```python
from build123d import *

# Parameters (mm, degrees)
SKETCH3_R           = 24
BOSS_EXTRUDE1_DEPTH = 19
BOSS_EXTRUDE2_DEPTH = 19
SKETCH7_R           = 8
BOSS_EXTRUDE3_DEPTH = 22.5
BOSS_EXTRUDE4_DEPTH = 26
SKETCH9_W           = 3
SKETCH9_H           = 19.17
BOSS_EXTRUDE5_DEPTH = 3.1
SKETCH10_R          = 1.68
CUT_EXTRUDE1_DEPTH  = 15
SKETCH11_R          = 21.7
CUT_EXTRUDE2_DEPTH  = 2
SKETCH12_R          = 12.95
SKETCH12_R_2        = 10.35
BOSS_EXTRUDE6_DEPTH = 2.06
SKETCH13_R          = 3.35
BOSS_EXTRUDE7_DEPTH = 10
BOSS_EXTRUDE8_DEPTH = 6.5


with BuildPart() as part:
    # Sketch3 → Boss-Extrude1 (new body)
    with BuildSketch(Plane.XY):
        with Locations((225, 142.5)):
            Circle(SKETCH3_R)
    extrude(amount=BOSS_EXTRUDE1_DEPTH)

    # Sketch5 → Boss-Extrude2 (add)
    with BuildSketch(Plane.XY):
        with BuildLine():
            Line((201, 142.5), (200.127626755, 106.785172639))
            Line((200.127626755, 106.785172639), (203.414220338, 106.785172639))
            Line((203.414220338, 106.785172639), (215.733540757, 120.361058447))
            ThreePointArc((215.733540757, 120.361058447), (205.020072299, 129.203290291), (201, 142.5))
        make_face()
    extrude(amount=BOSS_EXTRUDE2_DEPTH)

    # Sketch7 → Boss-Extrude3 (add)
    with BuildSketch(Plane(origin=(0, 128.5, 0), x_dir=(-1, 0, 0), z_dir=(0, -1, 0))):
        with Locations(Location((-233.969805688, -10, 0), (0, 0, 270))):
            Circle(SKETCH7_R)
    extrude(amount=BOSS_EXTRUDE3_DEPTH)

    # Sketch8 → Boss-Extrude4 (add)
    with BuildSketch(Plane(origin=(0, 158.5, 0), x_dir=(-1, 0, 0), z_dir=(0, -1, 0))):
        Polygon((-241.33102162, -5.75), (-241.33102162, -14.25), (-233.969805688, -18.5), (-226.608589756, -14.25), (-226.608589756, -5.75), (-233.969805688, -1.5), align=None)
    extrude(amount=-BOSS_EXTRUDE4_DEPTH)

    # Sketch9 → Boss-Extrude5 (add)
    with BuildSketch(Plane(origin=(197.401507206, -4.821745091, 0), x_dir=(0, 0, 1), z_dir=(-0.999701816720525, 0.024418796974499463, 0))):
        with Locations((20.5, 121.225206973)):
            Rectangle(SKETCH9_W, SKETCH9_H)
    extrude(amount=-BOSS_EXTRUDE5_DEPTH)

    # Sketch10 → Cut-Extrude1 (cut)
    with BuildSketch(Plane(origin=(197.401507206, -4.821745091, 0), x_dir=(0, 0, 1), z_dir=(-0.9997018167205249, 0.02441879697449946, 0))):
        with Locations(Location((3.14, 143.570206973, 0), (0, 0, 270))):
            Circle(SKETCH10_R)
        with BuildLine():
            Line((0, 119.880206973), (0, 115.990206973))
            Line((0, 115.990206973), (3.205, 115.990206973))
            ThreePointArc((3.205, 115.990206973), (5.15, 117.935206973), (3.205, 119.880206973))
            Line((3.205, 119.880206973), (0, 119.880206973))
        make_face()
        with BuildLine():
            Line((22, 115.990206973), (22, 119.880206973))
            Line((22, 119.880206973), (18.795, 119.880206973))
            ThreePointArc((18.795, 119.880206973), (16.85, 117.935206973), (18.795, 115.990206973))
            Line((18.795, 115.990206973), (22, 115.990206973))
        make_face()
    extrude(amount=-CUT_EXTRUDE1_DEPTH, mode=Mode.SUBTRACT)

    # Sketch11 → Cut-Extrude2 (cut)
    with BuildSketch(Plane.XY.offset(19)):
        with Locations((225, 142.5)):
            Circle(SKETCH11_R)
    extrude(amount=-CUT_EXTRUDE2_DEPTH, mode=Mode.SUBTRACT)

    # Sketch12 → Boss-Extrude6 (add)
    with BuildSketch(Plane.XY.offset(17)):
        with Locations((225, 142.5)):
            Circle(SKETCH12_R)
        with Locations((225, 142.5)):
            Circle(SKETCH12_R_2, mode=Mode.SUBTRACT)
    extrude(amount=BOSS_EXTRUDE6_DEPTH)

    # Sketch13 → Boss-Extrude7 (add)
    with BuildSketch(Plane.XY.offset(17)):
        with Locations((225, 138.9)):
            Circle(SKETCH13_R)
    extrude(amount=BOSS_EXTRUDE7_DEPTH)

    # Sketch14 → Boss-Extrude8 (add)
    with BuildSketch(Plane.XY.offset(17)):
        with BuildLine():
            Line((216.575, 142.25), (233.425, 142.25))
            ThreePointArc((233.425, 142.25), (234.5, 141.175), (233.425, 140.1))
            Line((233.425, 140.1), (216.575, 140.1))
            ThreePointArc((216.575, 140.1), (215.5, 141.175), (216.575, 142.25))
        make_face()
    extrude(amount=BOSS_EXTRUDE8_DEPTH)


solid = part.part
```
Build history of the part. All positions in model axes, mm. A direction names the side the tool comes from. Give positions to 0.01 mm unless a question says otherwise; leave off trailing zeros. Loops run counter-clockwise (first coordinate to the right, second up) from the corner with the lowest first, then second, coordinate; pieces in that order, holes last.
1) Probe line 1 along Y through (x, z) = (225, 18.45); line 2 along Y through (x, z) = (214.5, 18.5); line 3 along Y through (x, z) = (230.5, 18.25). List the from-to ranges inside material, lowest first.
Values follow:
line 1: y = 118.5 to 120.8, 129.55 to 132.15, 135.55 to 142.25, 152.85 to 155.45, 164.2 to 166.5
line 2: y = 119 to 123.51, 134.92 to 150.08, 161.49 to 164.08
line 3: y = 119.14 to 121.51, 130.78 to 133.73, 140.1 to 142.25, 151.27 to 154.22, 163.49 to 165.86
2) Band-saw the part on A-A on x = 218.5. List the corners of the cut face in (y, z).
Values follow:
outline: (119.4, 0) - (165.6, 0) - (165.6, 19) - (163.2, 19) - (163.2, 17) - (153.7, 17) - (153.7, 19.06) - (150.55, 19.06) - (150.55, 17) - (142.25, 17) - (142.25, 23.5) - (140.1, 23.5) - (140.1, 17) - (134.45, 17) - (134.45, 19.06) - (131.3, 19.06) - (131.3, 17) - (121.8, 17) - (121.8, 19) - (119.4, 19) - close
3) Band-saw the part on D-D on y = 130.5. List the corners of the cut face in (x, z), then the cut area to 3 significant figures.
Values follow:
outline: (200.71, 0) - (245.78, 0) - (245.78, 19) - (243.08, 19) - (243.08, 17) - (229.87, 17) - (229.87, 19.06) - (220.13, 19.06) - (220.13, 17) - (206.92, 17) - (206.92, 19) - (200.71, 19) - close
area: 804 mm2
4) Band-saw the part on C-C on z = 12.5. List the corners of the cut face in (x, y).
Values follow:
outline: (200.13, 106.79) - (203.41, 106.79) - (215.73, 120.36) arc R24 ccw to (226.37, 118.54) - (226.37, 106) - (241.57, 106) - (241.57, 125.14) arc R24 ccw to (241.33, 160.09) - (241.33, 184.5) - (226.61, 184.5) - (226.61, 166.45) arc R24 ccw to (201, 142.5) - close
5) Band-saw the part on B-B on y = 171.5. List the corners of the cut face in (x, z).
Values follow:
outline: (226.61, 5.75) - (233.97, 1.5) - (241.33, 5.75) - (241.33, 14.25) - (233.97, 18.5) - (226.61, 14.25) - close
6) 3-axis set-ups, long thin cutter, end or side, ignore diameter. For faces 1 (the face through (234.3, 133.2, 17)), 2 (the face through (204.23, 112.94, 5.15)), 3 (the face through (209.49, 113.48, 9.37)): which of +Z, -Z, +X, -X, +Y, -Y reach the whole face in a straight line?
Values follow:
face 1: +Z
face 2: -Z
face 3: +Z, -Z, -Y
7) Two-plate mould, pull along X, no slides. Class faces 4 (the face through (219, 140.1, 20)), 5 (the face through (202, 106.785, 9)), 6 (the face through (237.599, 172.123, 3.595)): released by +X, released by -X, zero draft, split by the parting line, or undercut.
Values follow:
face 4: undercut
face 5: zero draft
face 6: released by +X
8) Drop flat-ended pins along their axis: P1, Ø7, axis at y = 176.5, z = 10.5, coming from the -X side; P2, Ø8, axis at y = 138, z = 12.5, coming from the -X side; P3, Ø10, axis at x = 231.5, y = 145, coming from the +Z side; P4, Ø16.5, axis at x = 228.5, y = 146, coming from the +Z side. Give the stop position or say it passes through.
Values follow:
P1: stops at x = 226.61
P2: stops at x = 200.79
P3: stops at z = 23.5
P4: stops at z = 27
